Design review of the part shown in the three views and the two pictorial views. Dimensions are in mm from the part's minimum x, y and z. A direction names the side the tool comes from. Give positions to 0.01 mm unless a question says otherwise; leave off trailing zeros. Write each loop counter-clockwise with the first axis right and the second up, starting at its lowest first coordinate (ties: lowest second). Pieces come first, ordered by that corner, then holes. Notation, with made-up numbers: (16.5, -9.5) -> (65.5, -9.5) arc R24 cw to (65.5, 14.5) -> close; hole circle Ø9 at (-7.5, 87.25). An arc over 180 degrees is marked (long way). Return JSON: item names as keys, results as strings. Group by question number.
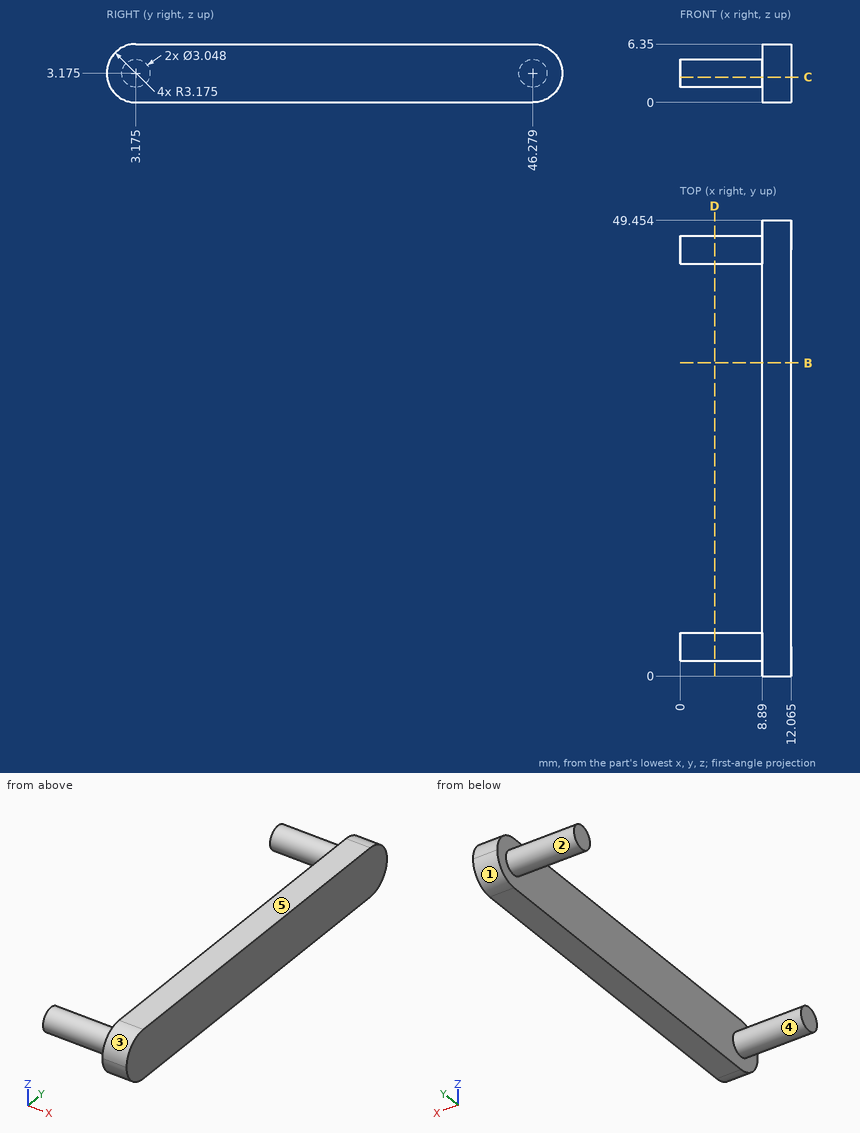
Q1. Tool access review of the marked faces 4 and 5: name each direction out of +Z, -Z, +X, -X, +Y, -Y from which nothing blocks a thin tool from reaching the whole face with its end or side.
Q2. Insertion check: pin 1 (3 mm diameter, centred on y = 36, z = 3, fed in from -X); pin 2 (3 mm diameter, centred on x = 9, z = 5, fed in from +Y). Each pin has a flat end and moves straight along its axis. Give the tip position at first contact, or say it passes through.
Q3. Take a section at B-B, the plane y = 34. Give the boundary of the cut face in (x, z) (3 decimals).
Q4. Take a section at D-D, the plane x = 3.75. Give the boundary of the cut face in (y, z) (1 decimal), plus the area to 3 significant figures.
Q5. For L1, parallel to Y at x = 7.5, z = 3 (1 decimal); L2, parallel to X at y = 14.5, z = 6 (3 decimals); L3, parallel to Y at x = 2.25, z = 2.75 (1 decimal), list the stretches that pass through material, from the lowest coordinate up. Write a range as from..to.
Q6. Take a section at C-C, the plane z = 2.75. Give the boundary of the cut face in (x, y) (1 decimal), plus the area to 3 significant figures.
Q7. Mouldability with a two-part tool opening along Y and no side actions: class the marked faces 1, 2 and 3 as +Y half, -Y half, draft (parallel to the pull), parting line (faces both ways), or undercut.
Final values:
{
 "1": {"face 4": "-X", "face 5": "+Z, +X, -X, +Y, -Y"},
 "2": {"pin 1": "stops at x = 8.89", "pin 2": "stops at y = 49.44"},
 "3": {"outline": "(8.89, 0) -> (12.065, 0) -> (12.065, 6.35) -> (8.89, 6.35) -> close"},
 "4": {"outline": "circle Ø3 at (3.2, 3.2); circle Ø3 at (46.3, 3.2)", "area": "14.6 mm²"},
 "5": {"L1": "y = 1.7..4.7, 44.8..47.8", "L2": "x = 8.89..12.065", "L3": "y = 1.7..4.6, 44.8..47.7"},
 "6": {"outline": "(0, 1.7) -> (8.9, 1.7) -> (8.9, 0) -> (12.1, 0) -> (12.1, 49.4) -> (8.9, 49.4) -> (8.9, 47.7) -> (0, 47.7) -> (0, 44.8) -> (8.9, 44.8) -> (8.9, 4.6) -> (0, 4.6) -> close", "area": "209 mm²"},
 "7": {"face 1": "+Y half", "face 2": "undercut", "face 3": "-Y half"}
}
